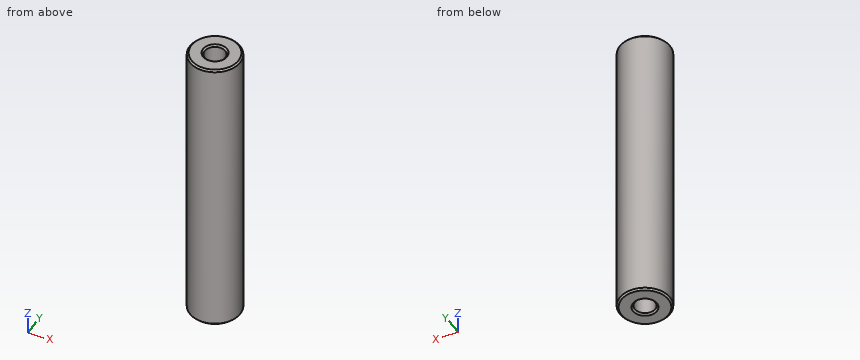
Autodesk Inventor part; units mm, degrees
ref_plane "YZ Plane" through (0, 0, 0) normal (1, 0, 0) x (0, 1, 0)
ref_plane "XZ Plane" through (0, 0, 0) normal (0, 1, 0) x (-1, 0, 0)
ref_plane "XY Plane" through (0, 0, 0) normal (0, 0, 1) x (1, 0, 0)
sketch "スケッチ1" plane through (0, 0, 0) normal (0, 0, 1) x (1, 0, 0)
  circle A0 centre (0, 0) radius 3
  dimension "d13" = 6
extrude "押し出し1" add sketch "スケッチ1" along normal mid plane 35
sketch "スケッチ2" plane through (0, 0, 17.5) normal (0, 0, 1) x (1, 0, 0)
  point P0 (0, 0)
  point P1 (0, 0)
hole "穴1" at (0, 0, 17.5) direction (0, 0, -1) diameter 2.459 depth 8.8 tip angle 118
mirror "ミラー1" about plane through (0, 0, 0) normal (0, 0, 1) of "穴1"
chamfer "面取り1" distance 0.2 angle 45 4 edges at (0, 1.2295, 17.5) (-3, 0, 17.5) (-3, 0, -17.5) (0, 1.2295, -17.5)
properties part number "ARF-330" material "鋼、炭素鋼"
Geometry: final body of the model. Coordinates: model frame, mm. Round coordinates to 2 decimals unless told otherwise and drop trailing zeros. Write each loop counter-clockwise with the first axis right and the second up, starting at its lowest first coordinate (ties: lowest second). Pieces come first, ordered by that corner, then holes. Notation, with made-up numbers: (53.5, 85) -> (82.5, 85) arc R26 cw to (82.5, 111) -> close; hole circle Ø7 at (12.5, 42). An arc over 180 degrees is marked (long way). Return JSON: item names as keys, results as strings.
Q1. First-contact query: pin 1 Ø2 at (x, y) = (0, 0) entering from -Z; pin 2 Ø1.5 at (x, y) = (0, 0) entering from -Z; pin 3 Ø1.5 at (x, z) = (1.5, 11) entering from +Y. Flat tips, straight axial feed; report the tip coordinate or a pass-through.
From the geometry:
{"pin 1": "z = -8.56", "pin 2": "z = -8.41", "pin 3": "y = 2.9"}
Q2. Section A-A on z = 10.5. Return the cut outline in (x, y).
From the geometry:
{"outline": "circle Ø6 at (0, 0); hole circle Ø2.46 at (0, 0)"}
Q3. Section B-B on z = 3.5. Return the cut outline in (x, y).
From the geometry:
{"outline": "circle Ø6 at (0, 0)"}
Q4. Ray query, line 1 (X direction, y = -0.05, z = -15); line 2 (Y direction, x = 0.1, z = 3). Return the intervals inside material, ascending.
From the geometry:
{"line 1": "-3 to -1.23, 1.23 to 3", "line 2": "-3 to 3"}
